Job drawing, mm, ordinate dimensions from the low corner. One solid piece. Coordinates: 2 decimals unless noted, no trailing zeros. Order: outer loops, then holes, each group sorted by start corner. A loop starts at its lowest first (then second) coordinate and runs counter-clockwise, first axis right, second up. Notation, with made-up numbers: (-15.75, -14) - (43.25, -14) arc R18 cw to (43.25, 6) - close; hole circle Ø4 at (-8, 28). An arc over 180 degrees is marked (long way). Use a Markdown table: item, result. Add a question column.
1) Wall check: L1, parallel to Y at x = 237.5, z = 7.5; L2, parallel to X at y = 13.25, z = 4.5; L3, parallel to X at y = 9.5, z = 8.25. Give the ranges that are in metal, low to high. Write a range as [from, to].
2) Two-plate mould, pull along X, no slides. Class the marked faces 1, 2, 3 and 4: +X half, -X half, draft (parallel to the pull), parting line (faces both ways), or undercut.
3) Saw through at C-C on z = 15.75. List the corners of the cut face in (x, y), then the cut area to 3 significant figures.
4) Saw through at B-B on x = 237.5. List the corners of the cut face in (y, z), then the cut area to 3 significant figures.
5) Saw through at A-A on y = 12.5. List the corners of the cut face in (x, z).
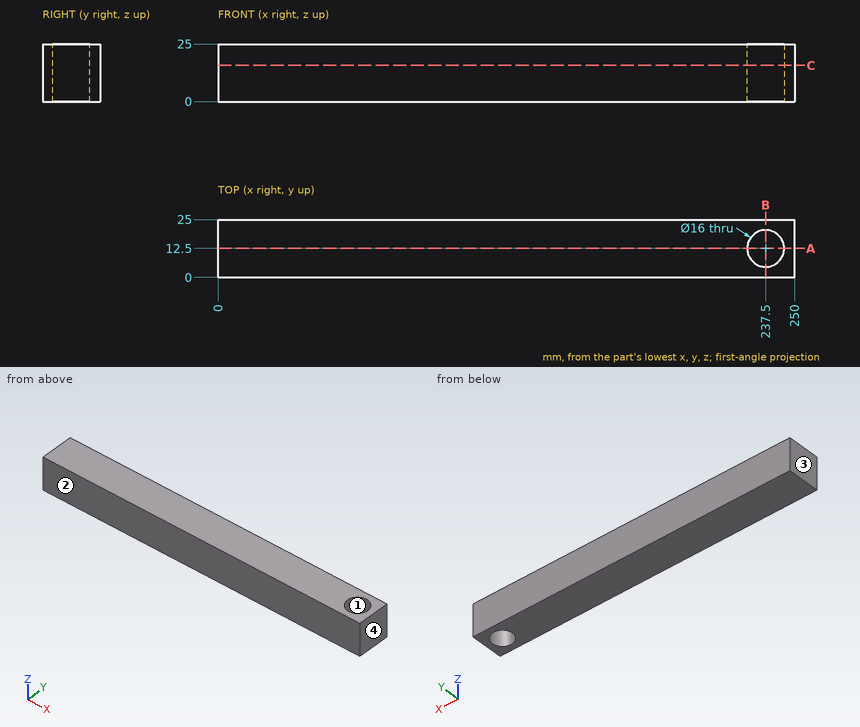
Results are:
| question | item | result |
|---|---|---|
| 1 | L1 | [0, 4.5], [20.5, 25] |
| 1 | L2 | [0, 229.54], [245.46, 250] |
| 1 | L3 | [0, 230.08], [244.92, 250] |
| 2 | face 1 | undercut |
| 2 | face 2 | draft |
| 2 | face 3 | -X half |
| 2 | face 4 | +X half |
| 3 | outline | (0, 0) - (250, 0) - (250, 25) - (0, 25) - close; hole circle Ø16 at (237.5, 12.5) |
| 3 | area | 6,050 mm2 |
| 4 | outline | (0, 0) - (4.5, 0) - (4.5, 25) - (0, 25) - close; (20.5, 0) - (25, 0) - (25, 25) - (20.5, 25) - close |
| 4 | area | 225 mm2 |
| 5 | outline | (0, 0) - (229.5, 0) - (229.5, 25) - (0, 25) - close; (245.5, 0) - (250, 0) - (250, 25) - (245.5, 25) - close |
